Geometry: see drawing. Coordinates: mm, zero at the bounding-box minimum. A direction names the side the tool comes from. Round coordinates to 2 decimals unless told otherwise and drop trailing zeros. Loops run counter-clockwise (first coordinate to the right, second up) from the corner with the lowest first, then second, coordinate; pieces in that order, holes last. Notation, with made-up numbers: (31.5, -39) - (88.5, -39) arc R21 ccw to (88.5, -34) - close; hole circle Ø10 at (62.5, 25). An arc over 180 degrees is marked (long way). One line per question, with ' | ' between items. Start each with the question number.
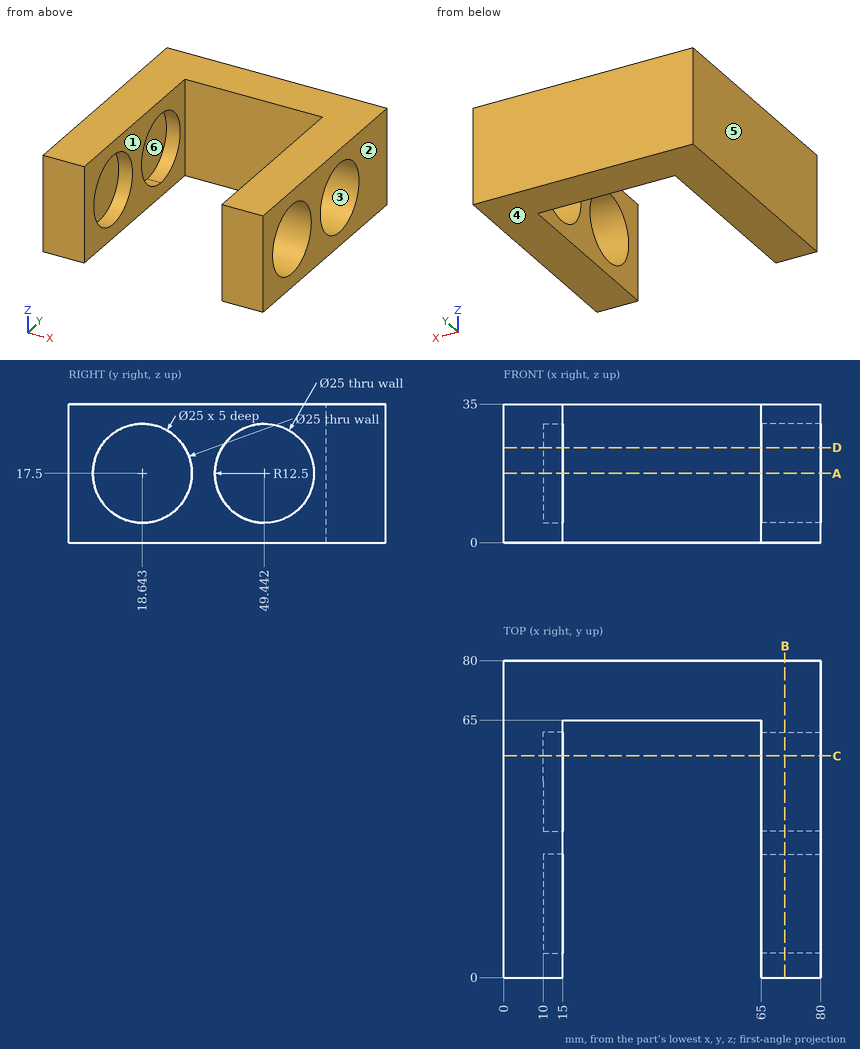
(1) Pull-direction query (Z, two-part tool) for the marked faces 4, 5 and 6; classes: released by +Z, released by -Z, zero draft, split by the parting line, or undercut.
(2) Section C-C, the plane y = 56. Output: boundary loops of the cut face in (x, z), plus the area to 3 significant figures.
(3) Section A-A, the plane z = 17.5. Output: boundary loops of the cut face in (x, y), plus the area to 3 significant figures.
(4) Section D-D, the plane z = 24. Output: boundary loops of the cut face in (x, y) (3 decimals), plus the area to 3 significant figures.
(5) Reachability of the marked faces 1, 2 and 3 from +Z, -Z, +X, -X, +Y, -Y: full face, straight path, thin tool, end or side. Return the list, or none.
(6) Section B-B, the plane x = 71. Output: boundary loops of the cut face in (y, z).
(7) Pin query (flat end, axial travel): P1, Ø4, axis at y = 47, z = 17.5, coming from the +X side; P2, Ø17.5, axis at x = 51.5, z = 9.5, coming from the -Y side. Return the tip coordinate at first contact, or that it passes through.
(8) Line query: line 1 along X through (y, z) = (13, 2.5); line 2 along Y through (x, z) = (68.5, 29) (1 decimal); line 3 along Y through (x, z) = (11.5, 24.5). Output: solid intervals per line, ascending. Write a range as from..to.
Derived:
1) face 4: released by -Z | face 5: zero draft | face 6: undercut
2) outline: (0, 0) - (15, 0) - (15, 6.86) - (10, 6.86) - (10, 28.14) - (15, 28.14) - (15, 35) - (0, 35) - close; (65, 0) - (80, 0) - (80, 6.86) - (65, 6.86) - close; (65, 28.14) - (80, 28.14) - (80, 35) - (65, 35) - close | area: 624 mm²
3) outline: (0, 0) - (15, 0) - (15, 6.14) - (10, 6.14) - (10, 31.14) - (15, 31.14) - (15, 36.94) - (10, 36.94) - (10, 61.94) - (15, 61.94) - (15, 65) - (65, 65) - (65, 61.94) - (80, 61.94) - (80, 80) - (0, 80) - close; (65, 0) - (80, 0) - (80, 6.14) - (65, 6.14) - close; (65, 31.14) - (80, 31.14) - (80, 36.94) - (65, 36.94) - close | area: 2,150 mm²
4) outline: (0, 0) - (15, 0) - (15, 7.966) - (10, 7.966) - (10, 29.32) - (15, 29.32) - (15, 38.765) - (10, 38.765) - (10, 60.119) - (15, 60.119) - (15, 65) - (65, 65) - (65, 60.119) - (80, 60.119) - (80, 80) - (0, 80) - close; (65, 0) - (80, 0) - (80, 7.966) - (65, 7.966) - close; (65, 29.32) - (80, 29.32) - (80, 38.765) - (65, 38.765) - close | area: 2,300 mm²
5) face 1: +Z, -Z, -Y | face 2: +Z, -Z, +X, +Y, -Y | face 3: +X
6) outline: (0, 0) - (80, 0) - (80, 35) - (0, 35) - close; hole circle Ø25 at (18.64, 17.5); hole circle Ø25 at (49.44, 17.5)
7) P1: stops at x = 10 | P2: stops at y = 65
8) line 1: x = 0..15, 65..80 | line 2: y = 0..13.7, 23.5..44.5, 54.3..80 | line 3: y = 0..8.29, 29..39.09, 59.8..80
